```python
from build123d import *

# Parameters (mm, degrees)
SKETCH1_W           = 25.4
SKETCH1_H           = 12.7
BOSS_EXTRUDE1_DEPTH = 50.8
CUT_EXTRUDE1_DEPTH  = 50.8
SKETCH3_W           = 50.8
SKETCH3_H           = 6.35
CUT_EXTRUDE3_DEPTH  = 59.198711326
SKETCH5_W           = 20.32
SKETCH5_H           = 45.72
CUT_EXTRUDE4_DEPTH  = 3.81


with BuildPart() as part:
    # Sketch1 → Boss-Extrude1 (new body)
    with BuildSketch(Plane.XY):
        with Locations((12.7, 6.35)):
            Rectangle(SKETCH1_W, SKETCH1_H)
    extrude(amount=-BOSS_EXTRUDE1_DEPTH)

    # Sketch2 → Cut-Extrude1 (cut)
    with BuildSketch(Plane.XY):
        with BuildLine():
            Line((8.509, 7.62), (16.891, 7.62))
            ThreePointArc((16.891, 7.62), (18.161, 6.35), (16.891, 5.08))
            Line((16.891, 5.08), (8.509, 5.08))
            ThreePointArc((8.509, 5.08), (7.239, 6.35), (8.509, 7.62))
        make_face()
    extrude(amount=-CUT_EXTRUDE1_DEPTH, mode=Mode.SUBTRACT)

    # Sketch3 → Cut-Extrude3 (cut, through all)
    with BuildSketch(Plane(origin=(25.4, 0, 0), x_dir=(0, 0, -1), z_dir=(1, 0, 0))):
        with Locations((25.4, 3.175)):
            Rectangle(SKETCH3_W, SKETCH3_H)
    extrude(amount=-CUT_EXTRUDE3_DEPTH, mode=Mode.SUBTRACT)

    # Sketch5 → Cut-Extrude4 (cut)
    with BuildSketch(Plane.XZ.offset(-7.62)):
        with Locations((12.7, -25.4)):
            Rectangle(SKETCH5_W, SKETCH5_H)
    extrude(amount=-CUT_EXTRUDE4_DEPTH, mode=Mode.SUBTRACT)


solid = part.part
```
Part model, mm, in its own coordinate system. A direction names the side the tool comes from. Round coordinates to 2 decimals unless told otherwise and drop trailing zeros. Order: outer loops, then holes, each group sorted by start corner. A loop starts at its lowest first (then second) coordinate and runs counter-clockwise, first axis right, second up. Notation, with made-up numbers: M 44.25,36.25 L 81.25,36.25 A23 cw 81.25,68.25 Z; hole C 7.5,64.25 d10. An arc over 180 degrees is marked long. Put each result on its own line as item: value. Start each with the question number.
1. Drill centre lines: probe 1 along Z at (x, y) = (12.25, 10.25); probe 2 along X at (y, z) = (9.25, -8); probe 3 along Y at (x, z) = (6.25, -43). Where is each one in solid material? Low to high. Write a range as [from, to].
2. Slice it at A-A on x = 19.5. List the corners of the cut face in (y, z).
3. Slice it at B-B on y = 9. List the corners of the cut face in (x, z).
4. Slice it at C-C on z = -11.5. List the corners of the cut face in (x, y).
5. Tool access for faces 4 (the face through (17.779, 7.258, -25.044)), 5 (the face through (4, 6.35, -25)), 6 (the face through (2.54, 9, -26)): list every direction of +Z, -Z, +X, -X, +Y, -Y with a clear straight run to the whole face (end or side of a thin tool).
6. Two-plate mould, pull along Y, no slides. Class faces 1 (the face through (13, 7.62, -50)), 2 (the face through (22.86, 9, -26)), 3 (the face through (13, 10, 0)): +Y half, -Y half, draft (parallel to the pull), parting line (faces both ways), or undercut.
7. Drop flat-ended pins along their axis: pin 1 (1.1 mm diameter, centred on x = 11.5, y = 9.5, fed in from +Z); pin 2 (0.8 mm diameter, centred on x = 13.5, z = -50, fed in from -Y). Give the stop position or say it passes through.
Findings:
1. probe 1: [-50.8, -48.26], [-2.54, 0]
1. probe 2: [0, 2.54], [22.86, 25.4]
1. probe 3: [6.35, 7.62], [11.43, 12.7]
2. outline: M 6.35,-50.8 L 12.7,-50.8 L 12.7,0 L 6.35,0 Z; hole M 7.62,-48.26 L 11.43,-48.26 L 11.43,-2.54 L 7.62,-2.54 Z
3. outline: M 0,-50.8 L 25.4,-50.8 L 25.4,0 L 0,0 Z; hole M 2.54,-48.26 L 22.86,-48.26 L 22.86,-2.54 L 2.54,-2.54 Z
4. outline: M 0,6.35 L 7.24,6.35 A1.27 cw 8.51,7.62 L 2.54,7.62 L 2.54,11.43 L 22.86,11.43 L 22.86,7.62 L 16.89,7.62 A1.27 cw 18.16,6.35 L 25.4,6.35 L 25.4,12.7 L 0,12.7 Z
5. face 4: +Z, -Z, -Y
5. face 5: +Z, -Z, +X, -X, -Y
5. face 6: none
6. face 1: -Y half
6. face 2: undercut
6. face 3: draft
7. pin 1: z = 0
7. pin 2: y = 7.62
